Job drawing, mm, ordinate dimensions from the low corner. One solid piece. A direction names the side the tool comes from. Give positions to 0.01 mm unless a question says otherwise; leave off trailing zeros. Write each loop counter-clockwise with the first axis right and the second up, starting at its lowest first coordinate (ties: lowest second). Pieces come first, ordered by that corner, then holes. Notation, with made-up numbers: M 26,-20 L 56,-20 A19 cw 56,-1 Z; hole C 89,0.25 d7. An arc over 180 degrees is marked long. Answer as CSV lines item,"result". Start each with the question number.
1) Slice it at A-A, the plane x = 9. Give the cut face in (y, z).
2) Slice it at D-D, the plane z = 3.5. Give the cut face in (x, y).
3) Pin check, flat tip, straight feed: pin 1 Ø0.8 at (x, y) = (9, 9) entering from -Z. Stop position of the tip, or through.
4) Wall check: line 1 along Y through (x, z) = (9, 1.4); line 2 along Y through (x, z) = (3, 2.5). Give the ranges that are in metal, low to high. Write a range as from..to.
5) Tool access for the marked faces 4, 5 and 6: list every direction of +Z, -Z, +X, -X, +Y, -Y with a clear straight run to the whole face (end or side of a thin tool).
6) Slice it at B-B, the plane z = 0.6. Give the cut face in (x, y).
7) Mould opens along Y. For the marked faces 1, 2 and 3 say: pulls with the +Y half, pulls with the -Y half, needs draft (parallel to the pull), parting line crosses it, or undercut.
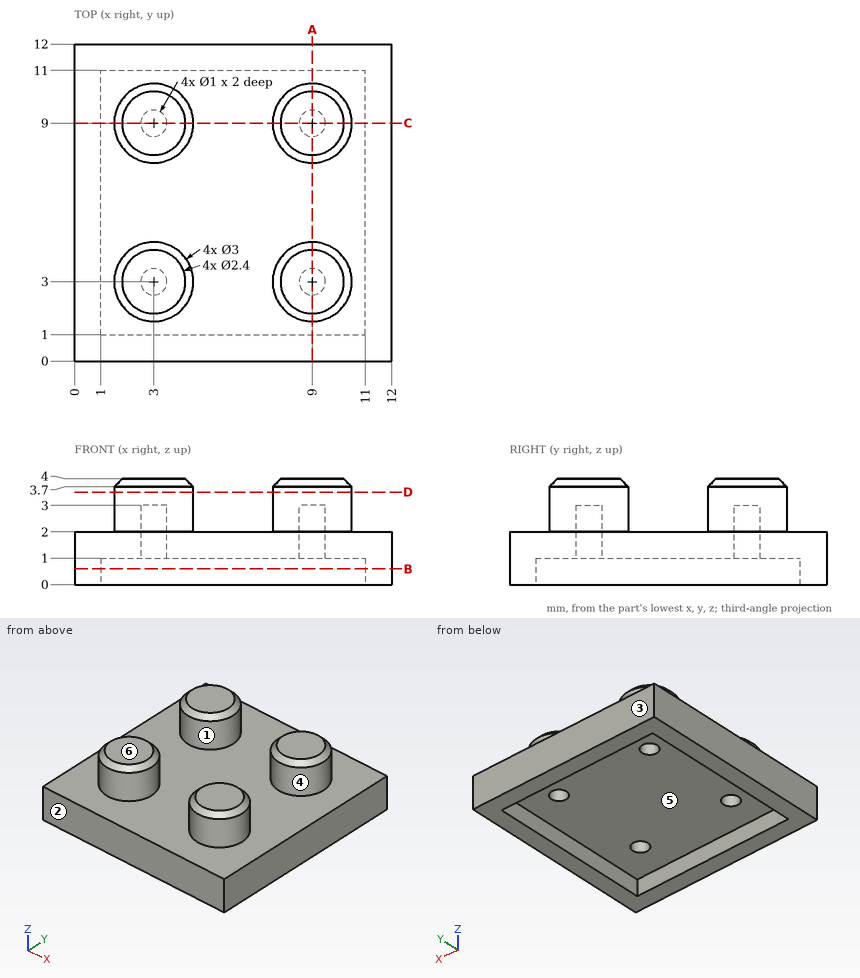
Found:
1,outline,"M 0,0 L 1,0 L 1,1 L 2.5,1 L 2.5,3 L 3.5,3 L 3.5,1 L 8.5,1 L 8.5,3 L 9.5,3 L 9.5,1 L 11,1 L 11,0 L 12,0 L 12,2 L 10.5,2 L 10.5,3.7 L 10.2,4 L 7.8,4 L 7.5,3.7 L 7.5,2 L 4.5,2 L 4.5,3.7 L 4.2,4 L 1.8,4 L 1.5,3.7 L 1.5,2 L 0,2 Z"
2,outline,"C 3,3 d3; C 3,9 d3; C 9,3 d3; C 9,9 d3"
3,pin 1,"z = 3"
4,line 1,"0..2.5, 3.5..8.5, 9.5..12"
4,line 2,"1.5..2.5, 3.5..4.5, 7.5..8.5, 9.5..10.5"
5,face 4,"+Z"
5,face 5,"-Z"
5,face 6,"+Z, +X, -X, +Y, -Y"
6,outline,"M 0,0 L 12,0 L 12,12 L 0,12 Z; hole M 1,1 L 11,1 L 11,11 L 1,11 Z"
7,face 1,"undercut"
7,face 2,"pulls with the -Y half"
7,face 3,"pulls with the +Y half"
